from build123d import *

# Parameters (mm, degrees)
SKETCH_1_W          = 118
SKETCH_1_H          = 55
SKETCH_1_R          = 1.6
EXTRUDE_1_DEPTH     = 3
SKETCH_2_R          = 1.5
CUT_EXTRUDE_1_DEPTH = 66.163256518
CUT_EXTRUDE_2_DEPTH = 66.163256518
FILLET_1_R          = 2
FILLET_2_R          = 3


with BuildPart() as part:
    # 草图1 → 凸台-拉伸1 (new body)
    with BuildSketch(Plane(origin=(0, 0, 0), x_dir=(1, 0, 0), z_dir=(0, 1, 0))):
        Rectangle(SKETCH_1_W, SKETCH_1_H)
        with Locations(Location((-55, 22.5, 0), (0, 0, 270))):
            Circle(SKETCH_1_R, mode=Mode.SUBTRACT)
        with Locations(Location((55, 22.5, 0), (0, 0, 270))):
            Circle(SKETCH_1_R, mode=Mode.SUBTRACT)
        with Locations(Location((-55, -22.5, 0), (0, 0, 270))):
            Circle(SKETCH_1_R, mode=Mode.SUBTRACT)
        with Locations(Location((55, -22.5, 0), (0, 0, 270))):
            Circle(SKETCH_1_R, mode=Mode.SUBTRACT)
        with Locations(Location((-18, 24, 0), (0, 0, 270))):
            Circle(SKETCH_1_R, mode=Mode.SUBTRACT)
        with Locations(Location((18, 24, 0), (0, 0, 270))):
            Circle(SKETCH_1_R, mode=Mode.SUBTRACT)
        with Locations(Location((18, -24, 0), (0, 0, 270))):
            Circle(SKETCH_1_R, mode=Mode.SUBTRACT)
        with Locations(Location((-18, -24, 0), (0, 0, 270))):
            Circle(SKETCH_1_R, mode=Mode.SUBTRACT)
    extrude(amount=EXTRUDE_1_DEPTH)

    # 草图2 → 切除-拉伸1 (cut, through all)
    with BuildSketch(Plane(origin=(0, 3, 0), x_dir=(1, 0, 0), z_dir=(0, 1, 0))):
        with Locations(Location((-37, 18, 0), (0, 0, 270))):
            Circle(SKETCH_2_R)
        with Locations(Location((37, 18, 0), (0, 0, 270))):
            Circle(SKETCH_2_R)
        with Locations(Location((37, -18, 0), (0, 0, 270))):
            Circle(SKETCH_2_R)
        with Locations(Location((-37, -18, 0), (0, 0, 270))):
            Circle(SKETCH_2_R)
    extrude(amount=-CUT_EXTRUDE_1_DEPTH, mode=Mode.SUBTRACT)

    # 草图3 → 切除-拉伸2 (cut, through all)
    with BuildSketch(Plane(origin=(0, 3, 0), x_dir=(1, 0, 0), z_dir=(0, 1, 0))):
        Polygon((-47, -11.850920072), (-9.867117107, 0), (-47, 11.850920072), align=None)
        Polygon((-37.132882893, 15), (0, 3.149079928), (37.132882893, 15), align=None)
        Polygon((9.867117107, 0), (47, -11.850920072), (47, 11.850920072), align=None)
        Polygon((-37.132882893, -15), (37.132882893, -15), (0, -3.149079928), align=None)
    extrude(amount=-CUT_EXTRUDE_2_DEPTH, mode=Mode.SUBTRACT)

    # 圆角1
    fillet_1_edges = [part.edges().sort_by_distance(p)[0] for p in [
        (47, 1.5, -11.850920072),
        (47, 1.5, 11.850920072),
        (9.867117107, 1.5, 0),
        (37.132882893, 1.5, -15),
        (0, 1.5, -3.149079928),
        (-37.132882893, 1.5, -15),
        (0, 1.5, 3.149079928),
        (37.132882893, 1.5, 15),
        (-37.132882893, 1.5, 15),
        (-9.867117107, 1.5, 0),
        (-47, 1.5, 11.850920072),
        (-47, 1.5, -11.850920072),
    ]]
    fillet(fillet_1_edges, radius=FILLET_1_R)

    # 圆角2
    fillet_2_edges = [part.edges().sort_by_distance(p)[0] for p in [
        (-59, 1.5, -27.5),
        (59, 1.5, -27.5),
        (59, 1.5, 27.5),
        (-59, 1.5, 27.5),
    ]]
    fillet(fillet_2_edges, radius=FILLET_2_R)


solid = part.part
Could you check a few things on this model? Use its own coordinates, in mm. A direction names the side the tool comes from. Give positions to 0.01 mm unless a question says otherwise; leave off trailing zeros. Order: outer loops, then holes, each group sorted by start corner. A loop starts at its lowest first (then second) coordinate and runs counter-clockwise, first axis right, second up. Notation, with made-up numbers: (-3, 32.25) -> (51, 32.25) arc R27 ccw to (51, 68.25) -> close; hole circle Ø6 at (75, 38). An arc over 180 degrees is marked (long way). Return JSON: item names as keys, results as strings.
1. Imagine slicing it at D-D on x = -18. List the corners of the cut face in (y, z) for me, then the cut area to 3 significant figures.
Answer list:
{"outline": "(0, -27.5) -> (3, -27.5) -> (3, -25.6) -> (0, -25.6) -> close; (0, -22.4) -> (3, -22.4) -> (3, -15) -> (0, -15) -> close; (0, -8.89) -> (3, -8.89) -> (3, -2.6) -> (0, -2.6) -> close; (0, 2.6) -> (3, 2.6) -> (3, 8.89) -> (0, 8.89) -> close; (0, 15) -> (3, 15) -> (3, 22.4) -> (0, 22.4) -> close; (0, 25.6) -> (3, 25.6) -> (3, 27.5) -> (0, 27.5) -> close", "area": "93.6 mm2"}
2. For pin 1 Ø5 at (x, z) = (-37, 18) entering from -Y, with a flat end and sliding along its axis, tell me the tip position at first contact or that it passes through.
Answer list:
{"pin 1": "stops at y = 0"}
3. Imagine slicing it at A-A on z = -18. List the corners of the cut face in (x, y) for me, then the cut area to 3 significant figures.
Answer list:
{"outline": "(-59, 0) -> (-38.5, 0) -> (-38.5, 3) -> (-59, 3) -> close; (-35.5, 0) -> (35.5, 0) -> (35.5, 3) -> (-35.5, 3) -> close; (38.5, 0) -> (59, 0) -> (59, 3) -> (38.5, 3) -> close", "area": "336 mm2"}
4. I need wall thicknesses on line 1 (X direction, y = 2.45, z = -22); line 2 (Z direction, x = -11, y = 2.45); line 3 (X direction, y = 2.25, z = -23.5). Which ranges of each line are inside material? Lowest first, please. Write a range as from..to.
Answer list:
{"line 1": "x = -59..-56.52, -53.48..53.48, 56.52..59", "line 2": "z = -27.5..-15, -6.66..6.66, 15..27.5", "line 3": "x = -59..-56.25, -53.75..-19.52, -16.48..16.48, 19.52..53.75, 56.25..59"}
5. On a 3-axis mill with a long thin cutter (end or side, diameter ignored), from which of +Z, -Z, +X, -X, +Y, -Y can I reach the whole of each face in a straight line? I mean faces 4 (the cylindrical face through (-14.446, 1.479, 0.035)), 5 (the flat face through (-59, 1, 0)). Say none if no direction works.
Answer list:
{"face 4": "+Y, -Y", "face 5": "+Z, -Z, -X, +Y, -Y"}
6. Imagine slicing it at B-B on x = -37. List the corners of the cut face in (y, z) for me, then the cut area to 3 significant figures.
Answer list:
{"outline": "(0, -27.5) -> (3, -27.5) -> (3, -19.5) -> (0, -19.5) -> close; (0, -16.5) -> (3, -16.5) -> (3, -8.66) -> (0, -8.66) -> close; (0, 8.66) -> (3, 8.66) -> (3, 16.5) -> (0, 16.5) -> close; (0, 19.5) -> (3, 19.5) -> (3, 27.5) -> (0, 27.5) -> close", "area": "95.0 mm2"}
7. Imagine slicing it at C-C on z = 12.5. List the corners of the cut face in (x, y) for me, then the cut area to 3 significant figures.
Answer list:
{"outline": "(-59, 0) -> (-26.22, 0) -> (-26.22, 3) -> (-59, 3) -> close; (26.22, 0) -> (59, 0) -> (59, 3) -> (26.22, 3) -> close", "area": "197 mm2"}
8. Thinking about a two-plate mould opening in Z: for faces 1 (the flat face through (-12.582, 1.521, 7.165)), 2 (the flat face through (-1, 1, 27.5)), 3 (the flat face through (-1, 1, -27.5)), which applies, pulls with the +Z half, pulls with the -Z half, needs draft (parallel to the pull), parting line crosses it, or undercut?
Answer list:
{"face 1": "undercut", "face 2": "pulls with the +Z half", "face 3": "pulls with the -Z half"}
